For this review, take the finished solid that the model builds, in its own axes (mm). A direction names the side the tool comes from. Give positions to 0.01 mm unless a question says otherwise; leave off trailing zeros. Loops run counter-clockwise (first coordinate to the right, second up) from the corner with the lowest first, then second, coordinate; pieces in that order, holes last. Notation, with made-up numbers: (-15.5, 46.5) - (3.5, 46.5) arc R21 cw to (3.5, 84.5) - close; hole circle Ø9 at (60, 58.25). An arc over 180 degrees is marked (long way). Answer as CSV lines item,"result".
from build123d import *

# Parameters (mm, degrees)
EXTRU_MINCE1_DEPTH      = 40
ENL_V_MAT_EXTRU_1_REACH = 107.282
ESQUISSE2_R             = 17.5
ENL_V_MAT_EXTRU_2_DEPTH = 146.129252737
ESQUISSE4_R             = 2.5
ENL_V_MAT_EXTRU_3_DEPTH = 146.129252737


with BuildPart() as part:
    # Esquisse1 → Extru.-Mince1 (new, symmetric)
    with BuildSketch(Plane.XY):
        with BuildLine():
            Line((-56.25, 82.5), (-56.25, 8))
            ThreePointArc((-56.25, 8), (-53.906854249, 2.343145751), (-48.25, 0))
            Line((-48.25, 0), (48.25, 0))
            ThreePointArc((48.25, 0), (53.906854249, 2.343145751), (56.25, 8))
            Line((56.25, 8), (56.25, 82.5))
            Line((56.25, 82.5), (53.25, 82.5))
            Line((53.25, 82.5), (53.25, 8))
            ThreePointArc((53.25, 8), (51.785533906, 4.464466094), (48.25, 3))
            Line((48.25, 3), (-48.25, 3))
            ThreePointArc((-48.25, 3), (-51.785533906, 4.464466094), (-53.25, 8))
            Line((-53.25, 8), (-53.25, 82.5))
            Line((-53.25, 82.5), (-56.25, 82.5))
        make_face()
    extrude(amount=EXTRU_MINCE1_DEPTH, both=True)

    # Esquisse2 → Enlèv. mat.-Extru.1 (cut, up to next)
    with BuildSketch(Plane(origin=(0, 3, 0), x_dir=(-1, 0, 0), z_dir=(0, 1, 0)), mode=Mode.PRIVATE) as enl_v_mat_extru_1_sk1:
        with Locations(Location((0, 0, 0), (0, 0, 90))):
            Circle(ESQUISSE2_R)
    enl_v_mat_extru_1_tool1 = extrude(enl_v_mat_extru_1_sk1.sketch, amount=-ENL_V_MAT_EXTRU_1_REACH, mode=Mode.PRIVATE) & part.part
    add(enl_v_mat_extru_1_tool1.solids().sort_by_distance((0, 3, 0))[0], mode=Mode.SUBTRACT)

    # Esquisse3 → Enlèv. mat.-Extru.2 (cut, through all)
    with BuildSketch(Plane(origin=(56.25, 0, 0), x_dir=(0, 0, -1), z_dir=(1, 0, 0))):
        with BuildLine():
            Line((-40, 41.241551833), (-21.084786145, 70.932490209))
            ThreePointArc((-21.084786145, 70.932490209), (-12.024719175, 79.418168919), (1.1e-07, 82.5))
            Line((1.1e-07, 82.5), (-40, 82.5))
            Line((-40, 82.5), (-40, 41.241551833))
        make_face()
        with BuildLine():
            Line((40, 82.5), (1.1e-07, 82.5))
            ThreePointArc((1.1e-07, 82.5), (12.024719271, 79.418168866), (21.084786145, 70.932490209))
            Line((21.084786145, 70.932490209), (40, 41.241551833))
            Line((40, 41.241551833), (40, 82.5))
        make_face()
    extrude(amount=-ENL_V_MAT_EXTRU_2_DEPTH, mode=Mode.SUBTRACT)

    # Esquisse4 → Enlèv. mat.-Extru.3 (cut, through all)
    with BuildSketch(Plane(origin=(56.25, 0, 0), x_dir=(0, 0, -1), z_dir=(1, 0, 0))):
        with Locations(Location((0, 57.5, 0), (0, 0, 90))):
            Circle(ESQUISSE4_R)
    extrude(amount=-ENL_V_MAT_EXTRU_3_DEPTH, mode=Mode.SUBTRACT)


solid = part.part
1) Wall thickness on line 1 (X direction, y = 47.5, z = -20); line 2 (Y direction, x = 1, z = 35.5); line 3 (X direction, y = 1, z = 0): over which ranges is each line inside the solid? List them lowest first. Write a range as from..to.
From the geometry:
line 1,"x = -56.25..-53.25, 53.25..56.25"
line 2,"y = 0..3"
line 3,"x = -52.12..-17.5, 17.5..52.12"
2) Insertion check: P1, Ø10, axis at y = 73.5, z = -29, coming from the +X side; P2, Ø10, axis at x = -42, z = -26.5, coming from the +Y side. Each pin has a flat end and moves straight along its axis. Give the tip position at first contact, or say it passes through.
From the geometry:
P1,"passes through"
P2,"stops at y = 3"
3) Machinability: for faces 1 (the cylindrical face through (-51.75, 4.43, 0.56)), 2 (the cylindrical face through (54.77, 59.81, -0.96)), which of the approach directions +Z, -Z, +X, -X, +Y, -Y give a long, thin tool a straight path to every point of the face, cutting with its end or side? Answer none if there is none.
From the geometry:
face 1,"+Z, -Z, +Y"
face 2,"+X, -X"
4) Draft analysis for pull direction X (two halves, no side actions). For faces 3 (the flat face through (54.771, 56.295, -30.41)), 4 (the cylindrical face through (53.844, 2.281, 0.56)), 5 (the cylindrical face through (51.82, 4.5, 0.56)), state which applies: pulls with the +X half, pulls with the -X half, needs draft (parallel to the pull), parting line crosses it, or undercut.
From the geometry:
face 3,"needs draft"
face 4,"pulls with the +X half"
face 5,"undercut"
5) Consider section B-B on z = -14.5. Write out the cut boundary in (x, y).
From the geometry:
outline,"(-56.25, 8) arc R8 ccw to (-48.25, 0) - (-9.8, 0) - (-9.8, 3) - (-48.25, 3) arc R5 cw to (-53.25, 8) - (-53.25, 77.87) - (-56.25, 77.87) - close; (9.8, 0) - (48.25, 0) arc R8 ccw to (56.25, 8) - (56.25, 77.87) - (53.25, 77.87) - (53.25, 8) arc R5 cw to (48.25, 3) - (9.8, 3) - close"
6) Consider section A-A on y = 29. Write out the cut boundary in (x, z), and give its area (3 significant figures).
From the geometry:
outline,"(-56.25, -40) - (-53.25, -40) - (-53.25, 40) - (-56.25, 40) - close; (53.25, -40) - (56.25, -40) - (56.25, 40) - (53.25, 40) - close"
area,"480 mm^2"
7) Consider section C-C on x = 0. Write out the cut boundary in (y, z).
From the geometry:
outline,"(0, -40) - (3, -40) - (3, -17.5) - (0, -17.5) - close; (0, 17.5) - (3, 17.5) - (3, 40) - (0, 40) - close"
8) Consider section D-D on y = 57.5. Write out the cut boundary in (x, z), and give its area (3 significant figures).
From the geometry:
outline,"(-56.25, -29.64) - (-53.25, -29.64) - (-53.25, -2.5) - (-56.25, -2.5) - close; (-56.25, 2.5) - (-53.25, 2.5) - (-53.25, 29.64) - (-56.25, 29.64) - close; (53.25, -29.64) - (56.25, -29.64) - (56.25, -2.5) - (53.25, -2.5) - close; (53.25, 2.5) - (56.25, 2.5) - (56.25, 29.64) - (53.25, 29.64) - close"
area,"326 mm^2"
